from build123d import *

# Parameters (mm, degrees)
SKETCH2_R           = 1
BOSS_EXTRUDE2_DEPTH = 2
FILLET1_R           = 2


with BuildPart() as part:
    # Sketch2 → Boss-Extrude2 (new body)
    with BuildSketch(Plane.XY):
        with BuildLine():
            Line((-3.823163379, 5.957240807), (-3.823163379, 7.694831843))
            ThreePointArc((-3.823163379, 7.694831843), (1.329416424, 7.130014771), (6.469831661, 7.796519188))
            Line((6.469831661, 7.796519188), (6.469831661, 14.872622199))
            Line((6.469831661, 14.872622199), (11.469831661, 14.872622199))
            Line((11.469831661, 14.872622199), (11.469831661, 9.743127337))
            Line((11.469831661, 9.743127337), (11.469831661, 5.993601449))
            ThreePointArc((11.469831661, 5.993601449), (3.825609616, 5.018374254), (-3.823163379, 5.957240807))
        make_face()
        with Locations((9.023220077, 8.376253999)):
            Circle(SKETCH2_R, mode=Mode.SUBTRACT)
        with Locations((9.016702167, 12.376248688)):
            Circle(SKETCH2_R, mode=Mode.SUBTRACT)
    extrude(amount=BOSS_EXTRUDE2_DEPTH)

    # Fillet1
    fillet1_edges = [part.edges().sort_by_distance(p)[0] for p in [
        (6.469831661, 7.796519188, 1),
        (6.469831661, 14.872622199, 1),
        (11.469831661, 14.872622199, 1),
        (11.469831661, 5.993601449, 1),
    ]]
    fillet(fillet1_edges, radius=FILLET1_R)


solid = part.part
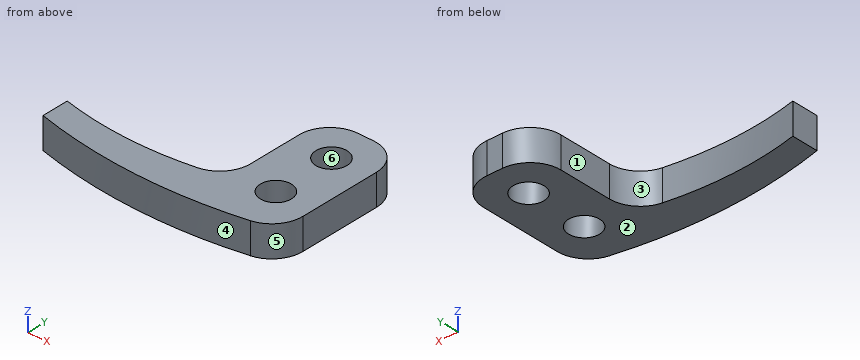
Geometry: final body of the model. Coordinates: model frame, mm. Face numbers are marked on the shaded views. A direction names the side the tool comes from. Give positions to 0.01 mm unless a question says otherwise; leave off trailing zeros. Order: outer loops, then holes, each group sorted by start corner. A loop starts at its lowest first (then second) coordinate and runs counter-clockwise, first axis right, second up. Notation, with made-up numbers: (18.5, 69) -> (57.5, 69) arc R7 cw to (57.5, 77) -> close; hole circle Ø1 at (60, -3.5). An arc over 180 degrees is marked (long way). Answer as a JSON object with one key per item and string values.
Q1. Draft query along X for the marked faces 4, 5 and 6. Return one class per face: released by +X, released by -X, zero draft, split by the parting line, or undercut.
Entries:
{"face 4": "split by the parting line", "face 5": "released by +X", "face 6": "undercut"}
Q2. Section A-A (x = 8.25). Output: boundary loops of the cut face in (y, z), plus the area to 3 significant figures.
Entries:
{"outline": "(5.35, 0) -> (7.74, 0) -> (7.74, 2) -> (5.35, 2) -> close; (9.01, 0) -> (11.73, 0) -> (11.73, 2) -> (9.01, 2) -> close; (13.02, 0) -> (14.86, 0) -> (14.86, 2) -> (13.02, 2) -> close", "area": "13.9 mm^2"}
Q3. Access query for the marked faces 1, 2 and 3. Directions: +Z, -Z, +X, -X, +Y, -Y. A direction counts if a zero-diameter tool reaches every point of the face in a straight line with its end or side. Return the directions, or none.
Entries:
{"face 1": "+Z, -Z, -X, +Y", "face 2": "-Z, +X, -X, +Y, -Y", "face 3": "+Z, -Z, +Y"}
Q4. Section D-D (y = 9.75). Output: boundary loops of the cut face in (x, z).
Entries:
{"outline": "(6.47, 0) -> (11.47, 0) -> (11.47, 2) -> (6.47, 2) -> close"}
Q5. Section C-C (z = 0.4). Output: boundary loops of the cut face in (x, y), plus the area to 3 significant figures.
Entries:
{"outline": "(-3.82, 5.96) arc R31.03 ccw to (9.86, 5.63) arc R2 ccw to (11.47, 7.59) -> (11.47, 12.87) arc R2 ccw to (9.47, 14.87) -> (8.47, 14.87) arc R2 ccw to (6.47, 12.87) -> (6.47, 9.42) arc R2 cw to (4.81, 7.44) arc R21.82 cw to (-3.82, 7.69) -> close; hole circle Ø2 at (9.02, 8.38); hole circle Ø2 at (9.02, 12.38)", "area": "60.3 mm^2"}
Q6. First-contact query: pin 1 (1.2 mm diameter, centred on x = 9.02, y = 12.38, fed in from +Z); pin 2 (0.6 mm diameter, centred on y = 10.5, z = 1, fed in from -X). Flat tips, straight axial feed; report the tip coordinate or a pass-through.
Entries:
{"pin 1": "passes through", "pin 2": "stops at x = 6.47"}
Q7. Section B-B (y = 8). Output: boundary loops of the cut face in (x, z).
Entries:
{"outline": "(5.88, 0) -> (8.1, 0) -> (8.1, 2) -> (5.88, 2) -> close; (9.95, 0) -> (11.47, 0) -> (11.47, 2) -> (9.95, 2) -> close"}
Q8. Material intervals for probe 1 along Y at (x, z) = (8.75, 1.05); probe 2 along X at (y, z) = (11.5, 1.6); probe 3 along X at (y, z) = (12.25, 0.45), sorted ascending.
Entries:
{"probe 1": "y = 5.42 to 7.41, 9.34 to 11.41, 13.34 to 14.87", "probe 2": "x = 6.47 to 8.53, 9.5 to 11.47", "probe 3": "x = 6.47 to 8.02, 10.01 to 11.47"}
